Geometry check sheet. Reference: the model listing, model coordinates, mm. Give positions to 0.01 mm unless a question says otherwise; leave off trailing zeros. Write each loop counter-clockwise with the first axis right and the second up, starting at its lowest first coordinate (ties: lowest second). Pieces come first, ordered by that corner, then holes.
(1) Cross-section at A-A (z = 0). Record the boundary of the cut face in (x, y).
(2) Cross-section at C-C (y = 220.5). Record the boundary of the cut face in (x, z).
(3) Thickness scan on line 1 along Y through (x, z) = (8, 0); line 2 along X through (y, z) = (100.5, 0.25); line 3 along Z through (x, y) = (-0.75, 379). Record the ranges inside material, lowest first.
(4) Cross-section at B-B (x = 4.75). Record the boundary of the cut face in (y, z).
(5) Depth check by flat-ended pin: P1, Ø5, axis at y = 169, z = -5.5, coming from the +X side; P2, Ø1.5, axis at y = 312, z = 5.5, coming from the +X side; P3, Ø4, axis at y = 390.034, z = 0, coming from the +X side; P4, Ø2, axis at y = 63.5, z = 2, coming from the +X side. Enter the tip coordinate at first touch or a pass-through.
```python
from build123d import *

# Parameters (mm, degrees)
SKETCH1_W               = 10
SKETCH1_H               = 399.034
SKETCH2_R               = 3.2
CUT_EXTRUDE1_DEPTH      = 11
CUT_EXTRUDE1_DEPTH_BACK = 11


with BuildPart() as part:
    # Sketch1 → Revolve2 (revolve)
    with BuildSketch(Plane(origin=(0, 0, 0), x_dir=(0, 0, -1), z_dir=(1, 0, 0))):
        with Locations((-5, 199.517)):
            Rectangle(SKETCH1_W, SKETCH1_H)
    revolve(axis=Axis((0, 0, 0), (0, 1, 0)))

    # Sketch2 → Cut-Extrude1 (cut, two sides)
    with BuildSketch(Plane(origin=(0, 0, 0), x_dir=(0, 0, -1), z_dir=(1, 0, 0))) as cut_extrude1_sk:
        with Locations((0, 390.034)):
            Circle(SKETCH2_R)
        with Locations((0, 12)):
            Circle(SKETCH2_R)
    extrude(amount=CUT_EXTRUDE1_DEPTH, mode=Mode.SUBTRACT)
    extrude(cut_extrude1_sk.sketch, amount=-CUT_EXTRUDE1_DEPTH_BACK, mode=Mode.SUBTRACT)


solid = part.part
```
Reply:
1. outline: (-10, 0) - (10, 0) - (10, 8.8) - (-10, 8.8) - close; (-10, 15.2) - (10, 15.2) - (10, 386.83) - (-10, 386.83) - close; (-10, 393.23) - (10, 393.23) - (10, 399.03) - (-10, 399.03) - close
2. outline: circle Ø20 at (0, 0)
3. line 1: y = 0 to 8.8, 15.2 to 386.83, 393.23 to 399.03
3. line 2: x = -10 to 10
3. line 3: z = -9.97 to 9.97
4. outline: (0, -8.8) - (399.03, -8.8) - (399.03, 8.8) - (0, 8.8) - close; hole circle Ø6.4 at (12, 0); hole circle Ø6.4 at (390.03, 0)
5. P1: stops at x = 9.54
5. P2: stops at x = 8.8
5. P3: passes through
5. P4: stops at x = 9.95
